```python
from build123d import *

# Parameters (mm, degrees)
SKETCH_1_R               = 1.55
EXTRUDE_1_DEPTH          = 2.2
HOLE_WIZARD_1_AT_2_COUNT = 2
HOLE_WIZARD_1_AT_2_PITCH = 21.360009363
HOLE_WIZARD_1_AT_3_COUNT = 2
HOLE_WIZARD_1_AT_3_PITCH = 15


with BuildPart() as part:
    # 草图1 → 凸台-拉伸1 (new body)
    with BuildSketch(Plane(origin=(0, 0, 0), x_dir=(0, 0, -1), z_dir=(1, 0, 0))):
        with BuildLine():
            Line((-16, 16.5), (-16, 13.5))
            ThreePointArc((-16, 13.5), (-17.05, 12.45), (-18.1, 13.5))
            Line((-18.1, 13.5), (-20, 13.5))
            Line((-20, 13.5), (-20, -13.5))
            Line((-20, -13.5), (-18.1, -13.5))
            ThreePointArc((-18.1, -13.5), (-17.05, -12.45), (-16, -13.5))
            Line((-16, -13.5), (-16, -16.5))
            Line((-16, -16.5), (-6, -16.5))
            Line((-6, -16.5), (-6, -13.5))
            ThreePointArc((-6, -13.5), (-4.95, -12.45), (-3.9, -13.5))
            Line((-3.9, -13.5), (3.9, -13.5))
            ThreePointArc((3.9, -13.5), (4.95, -12.45), (6, -13.5))
            Line((6, -13.5), (6, -16.5))
            Line((6, -16.5), (16, -16.5))
            Line((16, -16.5), (16, -13.5))
            ThreePointArc((16, -13.5), (17.05, -12.45), (18.1, -13.5))
            Line((18.1, -13.5), (20, -13.5))
            Line((20, -13.5), (20, 13.5))
            Line((20, 13.5), (18.1, 13.5))
            ThreePointArc((18.1, 13.5), (17.05, 12.45), (16, 13.5))
            Line((16, 13.5), (16, 16.5))
            Line((16, 16.5), (6, 16.5))
            Line((6, 16.5), (6, 13.5))
            ThreePointArc((6, 13.5), (4.95, 12.45), (3.9, 13.5))
            Line((3.9, 13.5), (-3.9, 13.5))
            ThreePointArc((-3.9, 13.5), (-4.95, 12.45), (-6, 13.5))
            Line((-6, 13.5), (-6, 16.5))
            Line((-6, 16.5), (-16, 16.5))
        make_face()
        with Locations((-10, -4.5)):
            Circle(SKETCH_1_R, mode=Mode.SUBTRACT)
        with Locations((-10, 10.5)):
            Circle(SKETCH_1_R, mode=Mode.SUBTRACT)
        with Locations((10, 3)):
            Circle(SKETCH_1_R, mode=Mode.SUBTRACT)
    extrude(amount=EXTRUDE_1_DEPTH)

    # 草图2 → 打孔尺寸(%根据十字)槽沉头木螺钉的类型1 (revolve, cut)
    with BuildSketch(Plane(origin=(2.2, 10.5, 10), x_dir=(0, 0, -1), z_dir=(0, 1, 0))):
        Polygon((0, 0), (0, 2.2), (1.55, 2.2), (1.55, 1.45), (3, 0), align=None)
    hole_wizard_1 = revolve(axis=Axis((8.55, 10.5, 10), (-1, 0, 0)), mode=Mode.SUBTRACT)

    # 打孔尺寸(%根据十字)槽沉头木螺钉的类型1 at 2: 打孔尺寸(%根据十字)槽沉头木螺钉的类型1 ×2
    with Locations(*[Vector(0, -0.3511234415883914, -0.9363291775690447) * (i * HOLE_WIZARD_1_AT_2_PITCH) for i in range(1, HOLE_WIZARD_1_AT_2_COUNT)]):
        add(hole_wizard_1, mode=Mode.SUBTRACT)

    # 打孔尺寸(%根据十字)槽沉头木螺钉的类型1 at 3: 打孔尺寸(%根据十字)槽沉头木螺钉的类型1 ×2
    with Locations(*[(0, -i * HOLE_WIZARD_1_AT_3_PITCH, 0) for i in range(1, HOLE_WIZARD_1_AT_3_COUNT)]):
        add(hole_wizard_1, mode=Mode.SUBTRACT)


solid = part.part
```
Check sheet for the modelled part. Datum: model origin and axes. Units: mm. A direction names the side the tool comes from. Give positions to 0.01 mm unless a question says otherwise; leave off trailing zeros. Loops run counter-clockwise (first coordinate to the right, second up) from the corner with the lowest first, then second, coordinate; pieces in that order, holes last. Notation, with made-up numbers: (-18, -25) - (37, -25) arc R26 ccw to (37, -7) - close; hole circle Ø10 at (80.5, 77). An arc over 180 degrees is marked (long way). One line per question, with ' | ' between items. Start each with the question number.
1. Draft check along Y on faces 1 (the conical face through (1, 9, 11)), 2 (the cylindrical face through (1.08, 12.45, 17.03)), 3 (the cylindrical face through (0.37, -3.45, 11.14)), 4 (the flat face through (1, -16.5, 11)). Enter one of: released by +Y, released by -Y, zero draft, split by the parting line, or undercut.
2. Cross-section at B-B, the plane y = -4.5. Enter the section's corners in (x, z), plus the area to 3 significant figures.
3. Material ranges on line 1 along Y through (x, z) = (0.3, 10); line 2 along Y through (x, z) = (0.45, -10); line 3 along Z through (x, y) = (0.2, -4.5), recorded low to high. Write a range as [from, to].
4. Cross-section at A-A, the plane z = 10. Enter the section's corners in (x, y), plus the area to 3 significant figures.
5. Gauge pin test, flat ends, axial feed: pin 1 Ø3.5 at (y, z) = (10.5, 10) entering from +X; pin 2 Ø0.6 at (x, z) = (1.5, 19) entering from +Y; pin 3 Ø0.7 at (x, y) = (1, -14.5) entering from -Z; pin 4 Ø3 at (y, z) = (-4.5, 10) entering from +X. Record the tip position at first contact, or that the pin passes through.
6. Cross-section at D-D, the plane x = 1.8. Give the number of separate pieces and of enclosed holes in the cut face, plus the area to 3 significant figures.
7. Set-up check for faces 5 (the flat face through (1, 13.5, 19)), 6 (the flat face through (1, -13.5, 19)), 7 (the flat face through (1, 15, -16)), 8 (the flat face through (1, -15, 6)): record each of +Z, -Z, +X, -X, +Y, -Y from which the full face is reachable in a straight line by a thin tool's end or side.
8. Cross-section at C-C, the plane z = -10. Enter the section's corners in (x, y).
Check result:
1) face 1: undercut | face 2: released by +Y | face 3: undercut | face 4: released by -Y
2) outline: (0, -20) - (2.2, -20) - (2.2, 7) - (0.75, 8.45) - (0, 8.45) - close; (0, 11.55) - (0.75, 11.55) - (2.2, 13) - (2.2, 20) - (0, 20) - close | area: 79.1 mm2
3) line 1: y = [-16.5, -6.05], [-2.95, 8.95], [12.05, 16.5] | line 2: y = [-16.5, 1.45], [4.55, 16.5] | line 3: z = [-20, 8.45], [11.55, 20]
4) outline: (0, -16.5) - (2.2, -16.5) - (2.2, -7.5) - (0.75, -6.05) - (0, -6.05) - close; (0, -2.95) - (0.75, -2.95) - (2.2, -1.5) - (2.2, 7.5) - (0.75, 8.95) - (0, 8.95) - close; (0, 12.05) - (0.75, 12.05) - (2.2, 13.5) - (2.2, 16.5) - (0, 16.5) - close | area: 54.8 mm2
5) pin 1: stops at x = 0.95 | pin 2: stops at y = 13.5 | pin 3: stops at z = -16 | pin 4: passes through
6) separate pieces: 1 | enclosed holes: 3 | area: 1,120 mm2
7) face 5: +Z, +X, -X, +Y | face 6: +Z, +X, -X, -Y | face 7: -Z, +X, -X, +Y | face 8: +X, -X, -Y
8) outline: (0, -16.5) - (2.2, -16.5) - (2.2, 0) - (0.75, 1.45) - (0, 1.45) - close; (0, 4.55) - (0.75, 4.55) - (2.2, 6) - (2.2, 16.5) - (0, 16.5) - close
